```python
from build123d import *

# Parameters (mm, degrees)
SKETCH1_W               = 200
SKETCH1_H               = 170
F_1_4_STEEL_PLATE_DEPTH = 6.35
SKETCH2_W               = 19.812
SKETCH2_H               = 6.604
BLADEHINGECUT_DEPTH     = 0.635
BLADEHINGEHOLE_D        = 3.556
SKETCH5_W               = 5.05
SKETCH5_H               = 5.05
BLADENUTCUT_DEPTH       = 2


with BuildPart() as part:
    # Sketch1 → 1/4" Steel Plate (new body)
    with BuildSketch(Plane(origin=(0, 0, 0), x_dir=(1, 0, 0), z_dir=(0, 1, 0))):
        Rectangle(SKETCH1_W, SKETCH1_H)
    extrude(amount=F_1_4_STEEL_PLATE_DEPTH)

    # Sketch2 → BladeHingeCut (cut)
    with BuildSketch(Plane(origin=(0, 6.35, 0), x_dir=(1, 0, 0), z_dir=(0, 1, 0))):
        with Locations((-80.188, -81.698)):
            Rectangle(SKETCH2_W, SKETCH2_H)
    bladehingecut = extrude(amount=-BLADEHINGECUT_DEPTH, mode=Mode.SUBTRACT)

    # BladeHingeHole (through all)
    with Locations(Plane(origin=(-74.473, 5.715, 81.698), x_dir=(0, 0, 1), z_dir=(0, 1, 0))):
        with Locations((0, 0), (0, -11.176)):
            bladehingehole = Hole(BLADEHINGEHOLE_D / 2)

    # Sketch5 → BladeNutCut (cut)
    with BuildSketch(Plane.XZ):
        with Locations((-85.649, 81.698)):
            Rectangle(SKETCH5_W, SKETCH5_H)
        with Locations((-74.473, 81.698)):
            Rectangle(SKETCH5_W, SKETCH5_H)
    bladenutcut = extrude(amount=-BLADENUTCUT_DEPTH, mode=Mode.SUBTRACT)

    # BladeHingeMirror: BladeHingeCut, BladeHingeHole, BladeNutCut across plane
    add(bladehingecut.mirror(Plane.ZY), mode=Mode.SUBTRACT)
    add(bladehingehole.mirror(Plane.ZY), mode=Mode.SUBTRACT)
    add(bladenutcut.mirror(Plane.ZY), mode=Mode.SUBTRACT)


solid = part.part
```
Part model, mm, in its own coordinate system. A direction names the side the tool comes from. Round coordinates to 2 decimals unless told otherwise and drop trailing zeros. Put each result on its own line as item: value. Start each with the question number.
1. Drill centre lines: probe 1 along Z at (x, y) = (75, 3); probe 2 along Z at (x, y) = (88, 6.25); probe 3 along Z at (x, y) = (75.5, 2.25). Where is each one in solid material? Low to high. Write a range as [from, to].
2. Two-plate mould, pull along Z, no slides. Class faces 4 (the face through (-1, 3, -85)), 5 (the face through (-76, 2, 83)), 6 (the face through (-1, 0, -1)): +Z half, -Z half, draft (parallel to the pull), parting line (faces both ways), or undercut.
3. Tool access for faces 1 (the face through (-80, 5.715, 82)), 2 (the face through (-1, 6.35, -1)), 3 (the face through (76, 2, 83)): list every direction of +Z, -Z, +X, -X, +Y, -Y with a clear straight run to the whole face (end or side of a thin tool).
4. Drop a flat-ended pin along its axis: pin 1 (4.5 mm diameter, centred on x = 85.649, z = 81.698, fed in from -Y). Give the stop position or say it passes through.
Findings:
1. probe 1: [-85, 80], [83.4, 85]
1. probe 2: [-85, 78.4]
1. probe 3: [-85, 80.25], [83.15, 85]
2. face 4: -Z half
2. face 5: undercut
2. face 6: draft
3. face 1: +Z, +Y
3. face 2: +Z, -Z, +X, -X, +Y
3. face 3: -Y
4. pin 1: y = 2
